Verification items for the finished model (mm, model axes). Give positions to 0.01 mm unless a question says otherwise; leave off trailing zeros. Write each loop counter-clockwise with the first axis right and the second up, starting at its lowest first coordinate (ties: lowest second). Pieces come first, ordered by that corner, then holes. Notation, with made-up numbers: M -16.75,19.5 L -12.75,19.5 A19 ccw -12.75,48.5 Z; hole C 46.25,-7 d1. An arc over 180 degrees is marked long. Answer as a JSON object with one key per item and string values.
Autodesk Inventor part; units mm, degrees
ref_plane "YZ Plane" through (0, 0, 0) normal (1, 0, 0) x (0, 1, 0)
ref_plane "XZ Plane" through (0, 0, 0) normal (0, 1, 0) x (-1, 0, 0)
ref_plane "XY Plane" through (0, 0, 0) normal (0, 0, 1) x (1, 0, 0)
sketch "Sketch1" plane through (0, 0, 0) normal (0, 1, 0) x (-1, 0, 0)
  line L0 (18.2419, 23.2079) -> (57.2419, 23.2079)
  line L1 (57.7419, 22.7079) -> (57.7419, -16.2921)
  line L2 (57.2419, -16.7921) -> (18.2419, -16.7921)
  line L3 (17.7419, -16.2921) -> (17.7419, 22.7079)
  line L4 (56.2419, 21.7079) -> (19.2419, 21.7079)
  line L5 (19.2419, 21.7079) -> (19.2419, -15.2921)
  line L6 (19.2419, -15.2921) -> (56.2419, -15.2921)
  line L7 (56.2419, -15.2921) -> (56.2419, 21.7079)
  arc A0 (18.2419, 23.2079) -> (17.7419, 22.7079) centre (18.2419, 22.7079) ccw
  arc A1 (57.7419, 22.7079) -> (57.2419, 23.2079) centre (57.2419, 22.7079) ccw
  arc A2 (57.2419, -16.7921) -> (57.7419, -16.2921) centre (57.2419, -16.2921) ccw
  arc A3 (17.7419, -16.2921) -> (18.2419, -16.7921) centre (18.2419, -16.2921) ccw
  point P0 (0, 0)
  point P1 (17.7419, 23.2079)
  point P2 (57.7419, 23.2079)
  point P3 (57.7419, -16.7921)
  dimension "d0" = 40
  dimension "d1" = 40
  dimension "d2" = 1.5
  dimension "d3" = 0.5
extrude "Extrusion1" add sketch "Sketch1" along normal blind 1906.45
sketch "Sketch2" plane through (-18.2419, 0, -16.7921) normal (0, 0, -1) x (-1, 0, 0)
  line L0 (0, 1906.45) -> (39, 1906.45)
  line L1 (19.5, 1906.45) -> (19.5, 0)
  line L2 (39, 0) -> (0, 0)
  circle A0 centre (19.5, 953.225) radius 5
  point P0 (-18.2419, 0)
  dimension "d6" = 10
extrude "Extrusion2" cut sketch "Sketch2" against normal blind 10
extrude "Extrusion3" cut sketch "Sketch2" against normal blind 231.3
properties part number "Metalon_Base_1"
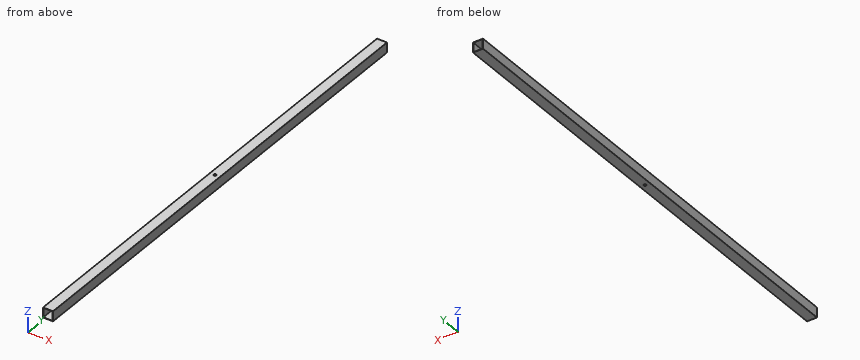
1) Go/stop test with a flat-tipped pin: pin 1 (6 mm diameter, centred on x = -45, z = 18.5, fed in from -Y). Record where the tip stops, or that it passes through.
Completed:
{"pin 1": "passes through"}
2) Thickness scan on L1, parallel to Z at x = -33, y = 1657; L2, parallel to X at y = 303, z = -9.5. Record the ranges inside material, lowest first.
Completed:
{"L1": "z = -16.79 to -15.29, 21.71 to 23.21", "L2": "x = -57.74 to -56.24, -19.24 to -17.74"}
3) Section check B-B on y = 1016. Record the boundary of the cut face in (x, z).
Completed:
{"outline": "M -57.74,-16.29 A0.5 ccw -57.24,-16.79 L -18.24,-16.79 A0.5 ccw -17.74,-16.29 L -17.74,22.71 A0.5 ccw -18.24,23.21 L -57.24,23.21 A0.5 ccw -57.74,22.71 Z; hole M -56.24,-15.29 L -19.24,-15.29 L -19.24,21.71 L -56.24,21.71 Z"}
4) Section check A-A on z = -3.5. Record the boundary of the cut face in (x, y), and give its area (3 significant figures).
Completed:
{"outline": "M -57.74,0 L -56.24,0 L -56.24,1906.45 L -57.74,1906.45 Z; M -19.24,0 L -17.74,0 L -17.74,1906.45 L -19.24,1906.45 Z", "area": "5,720 mm2"}
